Answer from the drawing. Dimensions are ordinates in mm from the lowest x, y and z of the part. Round coordinates to 2 decimals unless told otherwise and drop trailing zeros. Write each loop counter-clockwise with the first axis right and the second up, starting at its lowest first coordinate (ties: lowest second). Pieces come first, ordered by that corner, then holes. Notation, with made-up numbers: (41, 44.5) - (95, 44.5) arc R32 cw to (95, 81.5) - close; hole circle Ø3 at (-27.5, 88.5). An arc over 180 degrees is marked (long way). Answer as a JSON object with one key per item and string values.
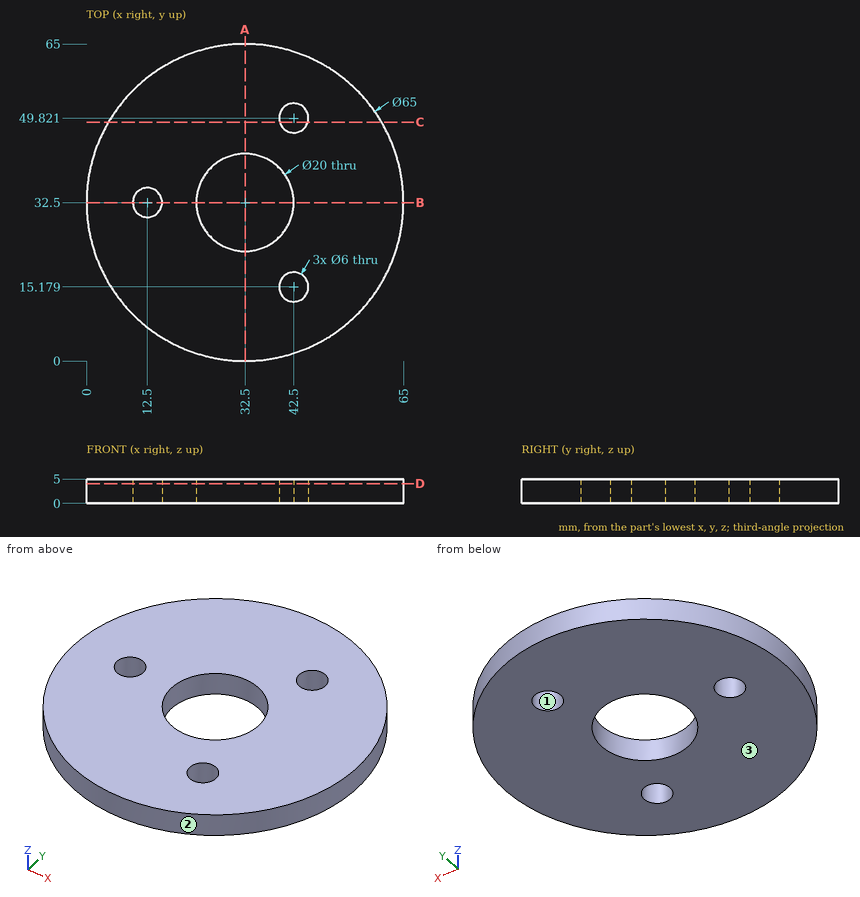
Item 1: A cutting plane is placed at A-A (x = 32.5). Write down the section's boundary in (y, z).
Results found:
{"outline": "(0, 0) - (22.5, 0) - (22.5, 5) - (0, 5) - close; (42.5, 0) - (65, 0) - (65, 5) - (42.5, 5) - close"}
Item 2: A cutting plane is placed at C-C (y = 49). Write down the section's boundary in (x, z) (1 decimal), and give its area (3 significant figures).
Results found:
{"outline": "(4.5, 0) - (39.6, 0) - (39.6, 5) - (4.5, 5) - close; (45.4, 0) - (60.5, 0) - (60.5, 5) - (45.4, 5) - close", "area": "251 mm²"}
Item 3: Each of these flat-tipped pins is pushed along its axis until it touches: P1, Ø1.5, axis at y = 12, z = 1.5, coming from the +X side; P2, Ø8, axis at x = 42.5, y = 15.18, coming from the +Z side; P3, Ø1, axis at x = 24.5, z = 2, coming from the -Y side; P4, Ø1.5, axis at y = 49, z = 2, coming from the -X side. Where does it stop, or does it pass through?
Results found:
{"P1": "x = 58.31", "P2": "z = 5", "P3": "y = 0.88", "P4": "x = 4.07"}
Item 4: Determine the mould class of the marked faces 1, 2 and 3 for opening direction Y: pulls with the +Y half, pulls with the -Y half, needs draft (parallel to the pull), parting line crosses it, or undercut.
Results found:
{"face 1": "undercut", "face 2": "parting line crosses it", "face 3": "needs draft"}
Item 5: Consider line 1 along Y through (x, z) = (32.5, 1.6); line 2 along X through (y, z) = (30, 0.25) (1 decimal); line 3 along Y through (x, z) = (45, 1) (1 decimal). Determine where each line is inside the solid, lowest interval first.
Results found:
{"line 1": "0 to 22.5, 42.5 to 65", "line 2": "0.1 to 10.8, 14.2 to 22.8, 42.2 to 64.9", "line 3": "2.5 to 13.5, 16.8 to 48.2, 51.5 to 62.5"}
Item 6: A cutting plane is placed at B-B (y = 32.5). Write down the section's boundary in (x, z).
Results found:
{"outline": "(0, 0) - (9.5, 0) - (9.5, 5) - (0, 5) - close; (15.5, 0) - (22.5, 0) - (22.5, 5) - (15.5, 5) - close; (42.5, 0) - (65, 0) - (65, 5) - (42.5, 5) - close"}
Item 7: A cutting plane is placed at D-D (z = 4.05). Write down the section's boundary in (x, y).
Results found:
{"outline": "circle Ø65 at (32.5, 32.5); hole circle Ø6 at (12.5, 32.5); hole circle Ø20 at (32.5, 32.5); hole circle Ø6 at (42.5, 15.18); hole circle Ø6 at (42.5, 49.82)"}
